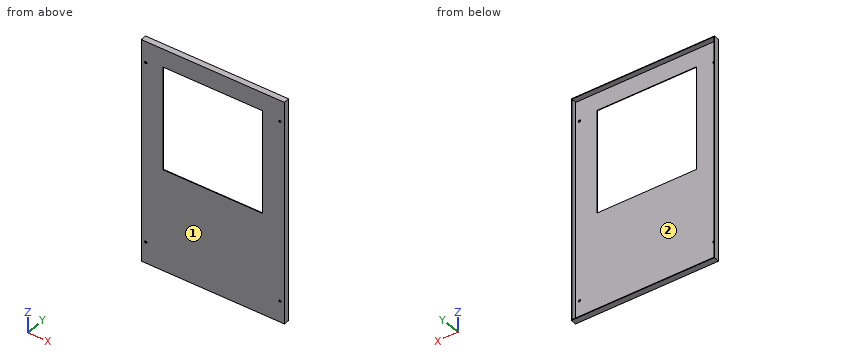
```python
from build123d import *

# Parameters (mm, degrees)
F0_W     = 622.3
F0_H     = 987.425
F0_R     = 4.7625
F0_W_2   = 431.8
F0_H_2   = 457.2
F1_DEPTH = 25.4
F2_T     = -2.54
F3_W     = 617.22
F3_H     = 22.86
F4_DEPTH = 982.345


with BuildPart() as f1:
    # F0 (on Front) → F1 (new body)
    with BuildSketch(Plane.XZ):
        with Locations((0, 493.7125)):
            Rectangle(F0_W, F0_H)
        with Locations((-292.1, 93.6625)):
            Circle(F0_R, mode=Mode.SUBTRACT)
        with Locations((292.1, 93.6625)):
            Circle(F0_R, mode=Mode.SUBTRACT)
        with Locations((-292.1, 893.7625)):
            Circle(F0_R, mode=Mode.SUBTRACT)
        with Locations((0, 678.66514)):
            Rectangle(F0_W_2, F0_H_2, mode=Mode.SUBTRACT)
        with Locations((292.1, 893.7625)):
            Circle(F0_R, mode=Mode.SUBTRACT)
    extrude(amount=F1_DEPTH)

    # F2
    f2_openings = [f1.faces().sort_by_distance(p)[0] for p in [
        (0, 0, 406.102773),
    ]]
    offset(amount=F2_T, openings=f2_openings, kind=Kind.INTERSECTION)

    # F3 (on face) → F4 (cut, through all)
    with BuildSketch(Plane.XY.offset(2.54)):
        with Locations((0, -11.43)):
            Rectangle(F3_W, F3_H)
    extrude(amount=F4_DEPTH, mode=Mode.SUBTRACT)


solid = f1.part
```
Can you work these out from the model? Positions are in its coordinate system, mm. Face numbers are marked on the shaded views. Round coordinates to 2 decimals unless told otherwise and drop trailing zeros. Loops run counter-clockwise (first coordinate to the right, second up) from the corner with the lowest first, then second, coordinate; pieces in that order, holes last. Notation, with made-up numbers: M 12,-16.75 L 27,-16.75 A12 cw 27,-8.75 Z; hole C 23,-29.5 d10. An arc over 180 degrees is marked long. Write item = value, one per line. Start each with the question number.
(1) I need wall thicknesses on line 1 along Z through (x, y) = (-292.1, -24.8) (3 decimals); line 2 along X through (y, z) = (-7.5, 807); line 3 along Z through (x, y) = (187.5, -4.5) (3 decimals). Which ranges of each line are inside material? Lowest first, please.
(2) Suppose I cut it at B-B on z = 852.5. Write out the boundary of the cut face in (x, y), plus the area to 3 significant figures.
(3) Suppose I cut it at A-A on x = 131. Write out the boundary of the cut face in (y, z) (3 decimals).
(4) Suppose I cut it at C-C on y = -4.5. Write out the boundary of the cut face in (x, z) (3 decimals), plus the area to 3 significant figures.
(5) Suppose I cut it at D-D on z = 77. Write out the boundary of the cut face in (x, y).
(6) If we mould it in two halves opening along Z, with no side actions, what happens to the marked faces 1 and 2? For each: released by +Z, released by -Z, zero draft, split by the parting line, or undercut.
(7) I'm going to push flat-ended pins straight in: P1, Ø3, axis at x = -1, y = -24, coming from the -Z side; P2, Ø11, axis at x = 292.1, z = 893.76, coming from the +Y side. Where does each tip first touch, or does it pass through?
Answer block:
q1.line_1 = 0 to 88.9, 98.425 to 889, 898.525 to 987.425
q1.line_2 = -311.15 to -308.61, 308.61 to 311.15
q1.line_3 = 0 to 2.54, 984.885 to 987.425
q2.outline = M -311.15,-25.4 L -215.9,-25.4 L -215.9,-22.86 L -308.61,-22.86 L -308.61,0 L -311.15,0 Z; M 215.9,-25.4 L 311.15,-25.4 L 311.15,0 L 308.61,0 L 308.61,-22.86 L 215.9,-22.86 Z
q2.area = 600 mm²
q3.outline = M -25.4,0 L 0,0 L 0,2.54 L -22.86,2.54 L -22.86,450.065 L -25.4,450.065 Z; M -25.4,907.265 L -22.86,907.265 L -22.86,984.885 L 0,984.885 L 0,987.425 L -25.4,987.425 Z
q4.outline = M -311.15,0 L 311.15,0 L 311.15,987.425 L -311.15,987.425 Z; hole M -308.61,2.54 L 308.61,2.54 L 308.61,984.885 L -308.61,984.885 Z
q4.area = 8,150 mm²
q5.outline = M -311.15,-25.4 L 311.15,-25.4 L 311.15,0 L 308.61,0 L 308.61,-22.86 L -308.61,-22.86 L -308.61,0 L -311.15,0 Z
q6.face_1 = zero draft
q6.face_2 = undercut
q7.P1 = 0
q7.P2 = -22.86
